from build123d import *

# Parameters (mm, degrees)
BOSS_EXTRUDE1_DEPTH = 5.5
SKETCH2_R           = 1.5
CUT_EXTRUDE1_DEPTH  = 5.5
SKETCH3_R           = 2.25
CUT_EXTRUDE2_DEPTH  = 4.25


with BuildPart() as part:
    # Sketch1 → Boss-Extrude1 (new body)
    with BuildSketch(Plane(origin=(0, 0, 0), x_dir=(1, 0, 0), z_dir=(0, 1, 0))):
        with BuildLine():
            Line((-3.124927795, 3.313350367), (0.875072205, 3.313350367))
            ThreePointArc((0.875072205, 3.313350367), (1.582178986, 3.020457148), (1.875072205, 2.313350367))
            Line((1.875072205, 2.313350367), (1.875072205, -1.686649633))
            ThreePointArc((1.875072205, -1.686649633), (1.582178986, -2.393756414), (0.875072205, -2.686649633))
            Line((0.875072205, -2.686649633), (-3.124927795, -2.686649633))
            ThreePointArc((-3.124927795, -2.686649633), (-3.832034576, -2.393756414), (-4.124927795, -1.686649633))
            Line((-4.124927795, -1.686649633), (-4.124927795, 2.313350367))
            ThreePointArc((-4.124927795, 2.313350367), (-3.832034576, 3.020457148), (-3.124927795, 3.313350367))
        make_face()
    extrude(amount=BOSS_EXTRUDE1_DEPTH)

    # Sketch2 → Cut-Extrude1 (cut)
    with BuildSketch(Plane(origin=(0, 5.5, 0), x_dir=(1, 0, 0), z_dir=(0, 1, 0))):
        with Locations(Location((-1.124927795, 0.313350367, 0), (0, 0, 270))):
            Circle(SKETCH2_R)
    extrude(amount=-CUT_EXTRUDE1_DEPTH, mode=Mode.SUBTRACT)

    # Sketch3 → Cut-Extrude2 (cut)
    with BuildSketch(Plane.XZ):
        with Locations(Location((-1.124927795, -0.313350367, 0), (0, 0, 270))):
            Circle(SKETCH3_R)
    extrude(amount=-CUT_EXTRUDE2_DEPTH, mode=Mode.SUBTRACT)


solid = part.part
Geometry: final body of the model. Coordinates: model frame, mm. A direction names the side the tool comes from. Give positions to 0.01 mm unless a question says otherwise; leave off trailing zeros. Write each loop counter-clockwise with the first axis right and the second up, starting at its lowest first coordinate (ties: lowest second). Pieces come first, ordered by that corner, then holes. Notation, with made-up numbers: (13, 31) -> (23, 31) arc R17 ccw to (23, 55) -> close; hole circle Ø1 at (50.25, 56.5). An arc over 180 degrees is marked (long way). Answer in a Markdown table with one row per item.
(1) Ray query, line 1 along Z through (x, y) = (0.6, 1.65); line 2 along Z through (x, y) = (-0.95, 2.35); line 3 along Y through (x, z) = (0.6, -1.2). Return the intervals inside material, ascending. Write a range as [from, to].
Answers below:
| item | result |
|---|---|
| line 1 | [-3.31, -1.76], [1.13, 2.69] |
| line 2 | [-3.31, -2.56], [1.93, 2.69] |
| line 3 | [4.25, 5.5] |
(2) Section query D-D on x = 0.6. Return loops of the section in (y, z).
Answers below:
| item | result |
|---|---|
| outline | (0, -3.31) -> (5.5, -3.31) -> (5.5, 2.69) -> (0, 2.69) -> (0, 1.13) -> (4.25, 1.13) -> (4.25, -1.76) -> (0, -1.76) -> close |
(3) Section query A-A on z = -1.5. Return loops of the section in (x, y), then the cut area to 3 significant figures.
Answers below:
| item | result |
|---|---|
| outline | (-4.12, 0) -> (-3.04, 0) -> (-3.04, 4.25) -> (-2.04, 4.25) -> (-2.04, 5.5) -> (-4.12, 5.5) -> close; (-0.21, 4.25) -> (0.79, 4.25) -> (0.79, 0) -> (1.88, 0) -> (1.88, 5.5) -> (-0.21, 5.5) -> close |
| area | 14.5 mm^2 |
(4) Draft query along X for faces 1 (the flat face through (-3, 4.25, -1)), 2 (the flat face through (-2, 0, 2)), 3 (the cylindrical face through (-1.7, 4.88, 1.07)), 4 (the cylindrical face through (-3.84, 2.71, -3.01)). Return one class per face: +X half, -X half, draft (parallel to the pull), parting line (faces both ways), or undercut.
Answers below:
| item | result |
|---|---|
| face 1 | undercut |
| face 2 | draft |
| face 3 | undercut |
| face 4 | -X half |
(5) Section query B-B on x = -2.2. Return loops of the section in (y, z).
Answers below:
| item | result |
|---|---|
| outline | (0, -3.31) -> (5.5, -3.31) -> (5.5, -1.36) -> (4.25, -1.36) -> (4.25, -2.29) -> (0, -2.29) -> close; (0, 1.66) -> (4.25, 1.66) -> (4.25, 0.73) -> (5.5, 0.73) -> (5.5, 2.69) -> (0, 2.69) -> close |
(6) Set-up query: faces 5 (the flat face through (0, 5.5, -2)), 6 (the cylindrical face through (1.106, 2.095, -0.02)). Return all of +Z, -Z, +X, -X, +Y, -Y with unobstructed straight access to the full face (end or side cutting, diameter ignored); none if empty.
Answers below:
| item | result |
|---|---|
| face 5 | +Z, -Z, +X, -X, +Y |
| face 6 | -Y |
(7) Section query C-C on y = 5. Return loops of the section in (x, z), then the cut area to 3 significant figures.
Answers below:
| item | result |
|---|---|
| outline | (-4.12, -2.31) arc R1 ccw to (-3.12, -3.31) -> (0.88, -3.31) arc R1 ccw to (1.88, -2.31) -> (1.88, 1.69) arc R1 ccw to (0.88, 2.69) -> (-3.12, 2.69) arc R1 ccw to (-4.12, 1.69) -> close; hole circle Ø3 at (-1.12, -0.31) |
| area | 28.1 mm^2 |
